Answer from the drawing. Dimensions are ordinates in mm from the lowest x, y and z of the part. A direction names the side the tool comes from. Coordinates: 2 decimals unless noted, no trailing zeros. Order: outer loops, then holes, each group sorted by start corner. A loop starts at its lowest first (then second) coordinate and runs counter-clockwise, first axis right, second up. Notation, with made-up numbers: (79.5, -36.75) -> (126.5, -36.75) arc R18 cw to (126.5, -15.75) -> close; hole circle Ø10 at (85.25, -3). An arc over 180 degrees is marked (long way). Use CSV: the item, a comma, the result in double quotes.
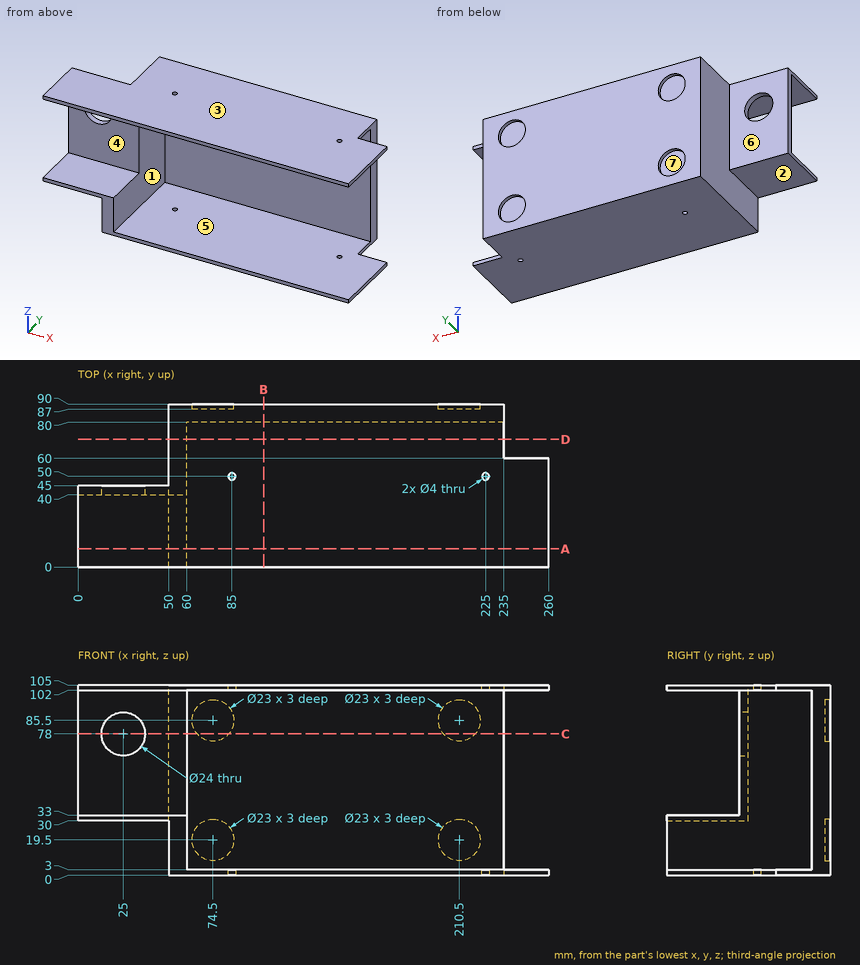
Item 1: The mould has two halves that part along Z. Classify the marked faces 1, 2 and 3: +Z half, -Z half, draft (parallel to the pull), parting line (faces both ways), or undercut.
Return value:
face 1,"undercut"
face 2,"-Z half"
face 3,"+Z half"
Item 2: Find section A-A, the plane y = 10. Give the vertices of the cut face in (x, z).
Return value:
outline,"(0, 30) -> (50, 30) -> (50, 0) -> (260, 0) -> (260, 3) -> (60, 3) -> (60, 33) -> (0, 33) -> close; (0, 102) -> (260, 102) -> (260, 105) -> (0, 105) -> close"
Item 3: A tool of negligible diameter and unlimited length cuts with its end or side. For the marked faces 4, 5, 6 and 7, from which of +Z, -Z, +X, -X, +Y, -Y can it reach the whole face along a straight path? Write none if from no direction.
Return value:
face 4,"+X, -X, -Y"
face 5,"+X, -Y"
face 6,"+Z, -Z, -X, +Y"
face 7,"+Y"
Item 4: Each of these flat-tipped pins is pushed along its axis until it touches: P1, Ø11.5, axis at x = 80, z = 81.5, coming from the +Y side; P2, Ø2.5, axis at x = 246, z = 103.5, coming from the +Y side; P3, Ø8, axis at x = 186.5, z = 31.5, coming from the -Y side; P4, Ø7, axis at x = 208, z = 22.5, coming from the +Y side. Where does it stop, or does it pass through?
Return value:
P1,"stops at y = 90"
P2,"stops at y = 60"
P3,"stops at y = 80"
P4,"stops at y = 87"
Item 5: Find section C-C, the plane z = 78. Give the vertices of the cut face in (x, y), then the cut area to 3 significant figures.
Return value:
outline,"(0, 40) -> (13, 40) -> (13, 45) -> (0, 45) -> close; (37, 40) -> (60, 40) -> (60, 80) -> (235, 80) -> (235, 90) -> (219.22, 90) -> (219.22, 87) -> (201.78, 87) -> (201.78, 90) -> (83.22, 90) -> (83.22, 87) -> (65.78, 87) -> (65.78, 90) -> (50, 90) -> (50, 45) -> (37, 45) -> close"
area,"2,280 mm^2"
Item 6: Straight lines are drawn through the part: line 1 along X through (y, z) = (87.7, 85.5); line 2 along Z through (x, y) = (74, 88); line 3 along Z through (x, y) = (212, 5.5). For each, find the intervals that lie inside material, in ascending order.
Return value:
line 1,"x = 50 to 63, 86 to 199, 222 to 235"
line 2,"z = 0 to 8.01, 30.99 to 74.01, 96.99 to 105"
line 3,"z = 0 to 3, 102 to 105"
Item 7: Find section B-B, the plane x = 102.5. Give the vertices of the cut face in (y, z).
Return value:
outline,"(0, 0) -> (90, 0) -> (90, 105) -> (0, 105) -> (0, 102) -> (80, 102) -> (80, 3) -> (0, 3) -> close"
Item 8: Find section D-D, the plane y = 70.5. Give the vertices of the cut face in (x, z).
Return value:
outline,"(50, 0) -> (235, 0) -> (235, 3) -> (60, 3) -> (60, 102) -> (235, 102) -> (235, 105) -> (50, 105) -> close"
